Verification items for the finished model (mm, model axes). Round coordinates to 2 decimals unless told otherwise and drop trailing zeros. Order: outer loops, then holes, each group sorted by start corner. A loop starts at its lowest first (then second) coordinate and runs counter-clockwise, first axis right, second up. Notation, with made-up numbers: (74, -4.5) -> (127, -4.5) arc R20 ccw to (127, 0.5) -> close; hole circle Ø1 at (84, -4.75). An arc over 180 degrees is marked (long way). Return JSON: item names as keys, results as strings. Group by question number.
1) Scan lines: L1, parallel to Y at x = -8.25, z = 0.3; L2, parallel to X at y = 14, z = 0.2; L3, parallel to Y at x = 40, z = 0.3. Record each from-to range of solid material in increasing order.
2) Section check A-A on x = 17. Enter the section's corners in (y, z).
3) Section check C-C on z = 0.6. State how many separate pieces and enclosed holes the cut face has, plus the area to 3 significant figures.
4) Section check D-D on y = 23.5. Enter the section's corners in (x, z).
5) Section check B-B on y = -10. Enter the section's corners in (x, z), plus the area to 3 significant figures.
```python
from build123d import *

# Parameters (mm, degrees)
BOARD_DEPTH    = 0.8
CUT_DEPTH      = 60.975412975
HOLESSKE_R     = 0.5
HOLESSKE_R_2   = 2.5
HOLES_DEPTH    = 60.975412975
HOLES2SKE_R    = 1
HOLES2_DEPTH   = 60.975412975
HOLES3SKE_R    = 0.5
HOLES3_DEPTH   = 60.975412975
HOLES4SKE_R    = 2.5
HOLES4SKE_R_2  = 0.5
HOLES4_DEPTH   = 60.975412975
FILLET1_R      = 1.8
SERVOSET_DEPTH = 10
FILLET2_R      = 0.6


with BuildPart() as part:
    # BoardSke → Board (new body)
    with BuildSketch(Plane.XY):
        with BuildLine():
            Line((42.5, 4.330127019), (-17.5, 38.97114317))
            ThreePointArc((-17.5, 38.97114317), (-22.5, 38.97114317), (-25, 34.641016151))
            Line((-25, 34.641016151), (-25, -34.641016151))
            ThreePointArc((-25, -34.641016151), (-22.5, -38.97114317), (-17.5, -38.97114317))
            Line((-17.5, -38.97114317), (42.5, -4.330127019))
            ThreePointArc((42.5, -4.330127019), (45, 0), (42.5, 4.330127019))
        make_face()
    extrude(amount=BOARD_DEPTH)

    # CutSke → Cut (cut, through all)
    with BuildSketch(Plane.XY.offset(0.8)):
        with BuildLine():
            Line((-7.973720558, 24.810889132), (-0.286612748, 11.496427842))
            ThreePointArc((-0.286612748, 11.496427842), (5.75, 9.959292144), (10.099504938, 5.5))
            Line((10.099504938, 5.5), (25.473720558, 5.5))
            Line((25.473720558, 5.5), (-7.973720558, 24.810889132))
        make_face()
        with BuildLine():
            Line((25.473720558, -5.5), (10.099504938, -5.5))
            ThreePointArc((10.099504938, -5.5), (5.75, -9.959292144), (-0.286612748, -11.496427842))
            Line((-0.286612748, -11.496427842), (-7.973720558, -24.810889132))
            Line((-7.973720558, -24.810889132), (25.473720558, -5.5))
        make_face()
    extrude(amount=-CUT_DEPTH, mode=Mode.SUBTRACT)

    # HolesSke → Holes (cut, through all)
    with BuildSketch(Plane.XY.offset(0.8)):
        with Locations((-6, 0)):
            Circle(HOLESSKE_R)
        with Locations((3, 5.196152423)):
            Circle(HOLESSKE_R)
        with Locations((3, -5.196152423)):
            Circle(HOLESSKE_R)
        Circle(HOLESSKE_R_2)
    extrude(amount=-HOLES_DEPTH, mode=Mode.SUBTRACT)

    # Holes2Ske → Holes2 (cut, through all)
    with BuildSketch(Plane.XY.offset(0.8)):
        with Locations((40, 0)):
            Circle(HOLES2SKE_R)
        with Locations((-20, -34.641016151)):
            Circle(HOLES2SKE_R)
        with Locations((-20, 34.641016151)):
            Circle(HOLES2SKE_R)
    extrude(amount=-HOLES2_DEPTH, mode=Mode.SUBTRACT)

    # Holes3Ske → Holes3 (cut, through all)
    with BuildSketch(Plane.XY.offset(0.8)):
        with Locations((40, 3)):
            Circle(HOLES3SKE_R)
        with Locations((40, -3)):
            Circle(HOLES3SKE_R)
        with Locations((-22.598076211, -33.141016151)):
            Circle(HOLES3SKE_R)
        with Locations((-17.401923789, -36.141016151)):
            Circle(HOLES3SKE_R)
        with Locations((-17.401923789, 36.141016151)):
            Circle(HOLES3SKE_R)
        with Locations((-22.598076211, 33.141016151)):
            Circle(HOLES3SKE_R)
    extrude(amount=-HOLES3_DEPTH, mode=Mode.SUBTRACT)

    # Holes4Ske → Holes4 (cut, through all)
    with BuildSketch(Plane.XY.offset(0.8)):
        with Locations((-8.25, 14.289419162)):
            Circle(HOLES4SKE_R)
        with Locations((-16.538942365, 14.044736682)):
            Circle(HOLES4SKE_R_2)
        with Locations((-16.538942365, 3.413610092)):
            Circle(HOLES4SKE_R_2)
        Polygon((-13.101840307, 8.209558145), (-13.101840307, 9.248788629), (-14.001840307, 9.768403872), (-14.901840307, 9.248788629), (-14.901840307, 8.209558145), (-14.001840307, 7.689942902), align=None)
    extrude(amount=-HOLES4_DEPTH, mode=Mode.SUBTRACT)

    # Fillet1
    fillet1_edges = [part.edges().sort_by_distance(p)[0] for p in [
        (25.473720558, 5.5, 0.4),
        (10.099504938, 5.5, 0.4),
        (-0.286612748, 11.496427842, 0.4),
        (-7.973720558, 24.810889132, 0.4),
        (25.473720558, -5.5, 0.4),
        (-7.973720558, -24.810889132, 0.4),
        (-0.286612748, -11.496427842, 0.4),
        (10.099504938, -5.5, 0.4),
    ]]
    fillet(fillet1_edges, radius=FILLET1_R)

    # ServoSetSke → ServoSet (cut)
    with BuildSketch(Plane.XY.offset(0.8)):
        Polygon((30.25, -5.155181486), (32, -5.155181486), (32, 6.344818514), (24, 6.344818514), (24, -5.155181486), (25.75, -5.155181486), (25.75, -7.355181486), (30.25, -7.355181486), align=None)
        Polygon((-15.75, -4), (-14, -4), (-14, -15.5), (-22, -15.5), (-22, -4), (-20.25, -4), (-20.25, -1.8), (-15.75, -1.8), align=None)
    extrude(amount=-SERVOSET_DEPTH, mode=Mode.SUBTRACT)

    # Fillet2
    fillet2_edges = [part.edges().sort_by_distance(p)[0] for p in [
        (32, 6.344818514, 0.4),
        (32, -5.155181486, 0.4),
        (30.25, -5.155181486, 0.4),
        (30.25, -7.355181486, 0.4),
        (25.75, -7.355181486, 0.4),
        (25.75, -5.155181486, 0.4),
        (24, -5.155181486, 0.4),
        (24, 6.344818514, 0.4),
        (-14, -4, 0.4),
        (-14, -15.5, 0.4),
        (-22, -15.5, 0.4),
        (-22, -4, 0.4),
        (-20.25, -4, 0.4),
        (-20.25, -1.8, 0.4),
        (-15.75, -1.8, 0.4),
        (-15.75, -4, 0.4),
    ]]
    fillet(fillet2_edges, radius=FILLET2_R)


solid = part.part
```
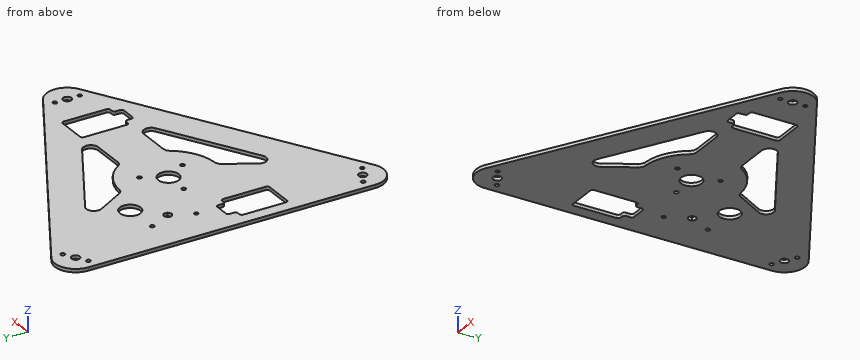
Check result:
{
 "1": {"L1": "-33.63 to 11.79, 16.79 to 33.63", "L2": "-25 to -17.04, -16.04 to -10.73, -5.77 to -1.73, 10.75 to 25.75", "L3": "-5.77 to -3.5, -2.5 to -1, 1 to 2.5, 3.5 to 5.77"},
 "2": {"outline": "(-19.05, 0) -> (-10.39, 0) -> (-10.39, 0.8) -> (-19.05, 0.8) -> close; (-5.5, 0) -> (5.5, 0) -> (5.5, 0.8) -> (-5.5, 0.8) -> close; (10.39, 0) -> (19.05, 0) -> (19.05, 0.8) -> (10.39, 0.8) -> close"},
 "3": {"separate pieces": "1", "enclosed holes": "21", "area": "2,600 mm^2"},
 "4": {"outline": "(-25, 0) -> (9.3, 0) -> (9.3, 0.8) -> (-25, 0.8) -> close"},
 "5": {"outline": "(-25, 0) -> (-22, 0) -> (-22, 0.8) -> (-25, 0.8) -> close; (-14, 0) -> (5.68, 0) -> (5.68, 0.8) -> (-14, 0.8) -> close; (17.68, 0) -> (32.68, 0) -> (32.68, 0.8) -> (17.68, 0.8) -> close", "area": "30.1 mm^2"}
}
